CAD build for the part. Positions are in the model's coordinates, mm. A direction names the side the tool comes from. Round coordinates to 2 decimals unless told otherwise and drop trailing zeros. Loops run counter-clockwise (first coordinate to the right, second up) from the corner with the lowest first, then second, coordinate; pieces in that order, holes last. Notation, with made-up numbers: M 0,14.5 L 52,14.5 A16 cw 52,23.5 Z; hole C -21,86.5 d8. An arc over 180 degrees is marked long. Put each result on its own line as item: value. Start each with the question number.
from build123d import *

# Parameters (mm, degrees)
F0_W    = 2.25
F0_H    = 6
F0_H_2  = 8
F2_SIZE = 0.25
F3_SIZE = 0.25
F4_R    = 10
F5_R    = 5


with BuildPart() as f1:
    # F0 (on Front) → F1 (revolve)
    with BuildSketch(Plane.XZ):
        with Locations((-3.425, 15)):
            Rectangle(F0_W, F0_H)
        Polygon((-6.35, 8), (-4.1, 8), (-2.3, 12), (-4.55, 12), align=None)
        with Locations((-5.225, 4)):
            Rectangle(F0_W, F0_H_2)
    revolve(axis=Axis((0, 0, 11.346421), (0, 0, -1)))

    # F2
    f2_edges = [f1.edges().sort_by_distance(p)[0] for p in [
        (6.35, 0, 0),
        (4.1, 0, 0),
    ]]
    chamfer(f2_edges, length=F2_SIZE)

    # F3
    f3_edges = [f1.edges().sort_by_distance(p)[0] for p in [
        (2.3, 0, 18),
        (4.55, 0, 18),
    ]]
    chamfer(f3_edges, length=F3_SIZE)

    # F4
    f4_edges = [f1.edges().sort_by_distance(p)[0] for p in [
        (4.55, 0, 12),
    ]]
    fillet(f4_edges, radius=F4_R)

    # F5
    f5_edges = [f1.edges().sort_by_distance(p)[0] for p in [
        (6.35, 0, 8),
    ]]
    fillet(f5_edges, radius=F5_R)


solid = f1.part
(1) Drill centre lines: line 1 along Y through (x, z) = (0, 16.25); line 2 along X through (y, z) = (-0.75, 16.25). Where is each one in solid material? Low to high.
(2) Tool access for faces 1 (the cylindrical face through (-4.203, -1.743, 15.973)), 2 (the flat face through (-2, -2, 18)), 3 (the cylindrical face through (0.534, 4.065, 4.179)): list every direction of +Z, -Z, +X, -X, +Y, -Y with a clear straight run to the whole face (end or side of a thin tool).
(3) Cut at A-A on z = 16.5. List the corners of the cut face in (x, y), and give its area (3 significant figures).
(4) Cut at B-B on z = 9.25. List the corners of the cut face in (x, y) (1 decimal), and give its area (3 significant figures).
(5) Mould opens along X. For faces 4 (the cylindrical face through (1.825, -1.4, 14.915)), 5 (the flat face through (-4, -3, 0)), 6 (the cylindrical face through (-6.057, 1.907, 3.635)) say: +X half, -X half, draft (parallel to the pull), parting line (faces both ways), or undercut.
(6) Flat gauge pins, fed straight in: pin 1 Ø4 at (y, z) = (0, 14) entering from -X; pin 2 Ø3 at (y, z) = (-3, 3) entering from -X; pin 3 Ø1 at (x, y) = (-1, -2.5) entering from -Z. Where does each tip first touch, or does it go through?
Taken from the geometry:
1. line 1: -4.55 to -2.3, 2.3 to 4.55
1. line 2: -4.49 to -2.17, 2.17 to 4.49
2. face 1: +Z
2. face 2: +Z, +X, -X, +Y, -Y
2. face 3: -Z
3. outline: C 0,0 d9.1; hole C 0,0 d4.6
3. area: 48.4 mm2
4. outline: C 0,0 d11.6; hole C 0,0 d7.1
4. area: 65.9 mm2
5. face 4: undercut
5. face 5: draft
5. face 6: parting line
6. pin 1: x = -4.78
6. pin 2: x = -6.17
6. pin 3: z = 10.02
